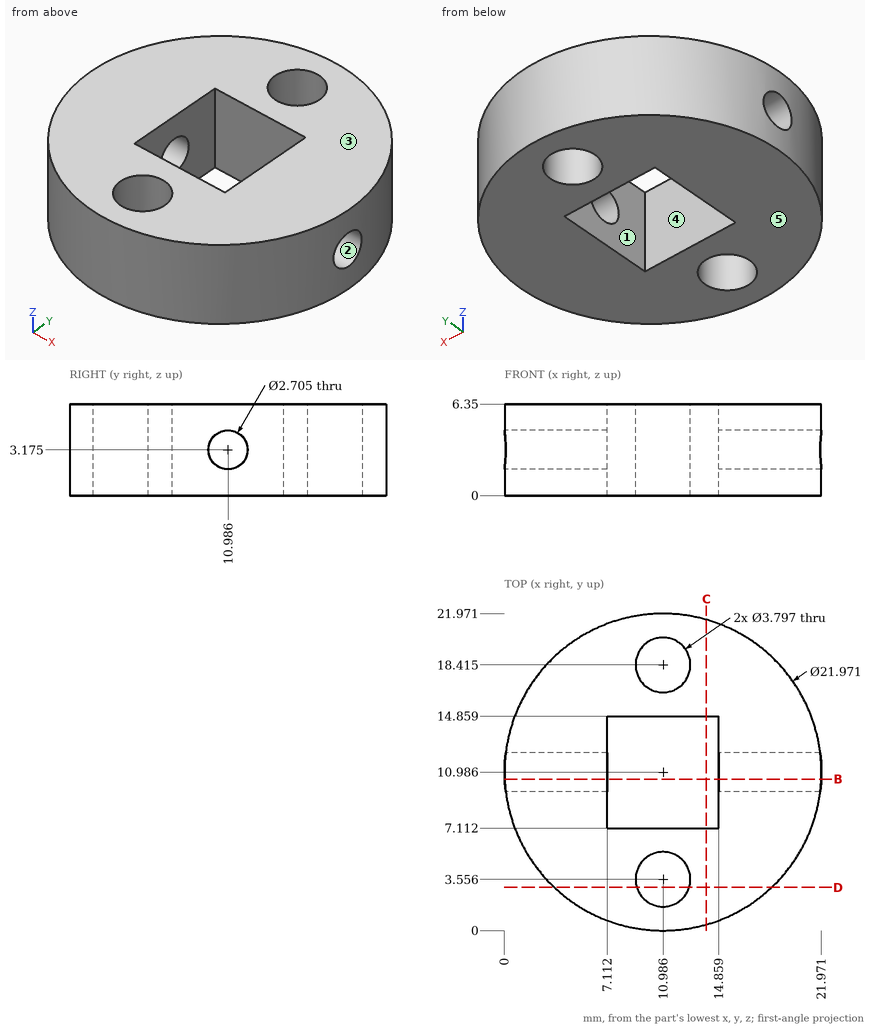
Input: dimensioned drawing with shaded views. Units: mm. Origin: part minimum x, y, z. A direction names the side the tool comes from. Coordinates: 2 decimals unless noted, no trailing zeros. Write each loop counter-clockwise with the first axis right and the second up, starting at its lowest first coordinate (ties: lowest second). Pieces come first, ordered by that corner, then holes. Notation, with made-up numbers: M 36,-18.75 L 72,-18.75 A11 ccw 72,-14.75 Z; hole C -19.75,60 d8. An arc over 180 degrees is marked long. Answer as CSV lines item,"result". Start each with the question number.
Q1. Reachability of the marked faces 4 and 5 from +Z, -Z, +X, -X, +Y, -Y: full face, straight path, thin tool, end or side. Return the list, or none.
Q2. Mould query, pull axis Z, two halves, no side actions, for the marked faces 1, 2 and 3. Classes: released by +Z, released by -Z, zero draft, split by the parting line, or undercut.
Q3. Cut plane B-B on y = 10.5. Return the cut outline in (x, z).
Q4. Cut plane C-C on x = 14. Return the cut outline in (y, z).
Q5. Cut plane D-D on y = 3. Return the cut outline in (x, z).
Q6. Line query: line 1 (Y direction, x = 11, z = 0.5) (1 decimal); line 2 (Y direction, x = 9.5, z = 6) (1 decimal); line 3 (Y direction, x = 13.75, z = 1) (1 decimal). Output: solid intervals per line, ascending. Write a range as from..to.
Findings below:
1,face 4,"+Z, -Z"
1,face 5,"-Z, +X, -X, +Y, -Y"
2,face 1,"zero draft"
2,face 2,"undercut"
2,face 3,"released by +Z"
3,outline,"M 0.01,0 L 7.11,0 L 7.11,1.91 L 0.01,1.91 Z; M 0.01,4.44 L 7.11,4.44 L 7.11,6.35 L 0.01,6.35 Z; M 14.86,0 L 21.96,0 L 21.96,1.91 L 14.86,1.91 Z; M 14.86,4.44 L 21.96,4.44 L 21.96,6.35 L 14.86,6.35 Z"
4,outline,"M 0.42,0 L 7.11,0 L 7.11,6.35 L 0.42,6.35 Z; M 14.86,0 L 21.55,0 L 21.55,6.35 L 14.86,6.35 Z"
5,outline,"M 3.44,0 L 9.17,0 L 9.17,6.35 L 3.44,6.35 Z; M 12.8,0 L 18.53,0 L 18.53,6.35 L 12.8,6.35 Z"
6,line 1,"y = 0..1.7, 5.5..7.1, 14.9..16.5, 20.3..22"
6,line 2,"y = 0.1..2.4, 4.7..7.1, 14.9..17.2, 19.6..21.9"
6,line 3,"y = 0.4..7.1, 14.9..21.6"
